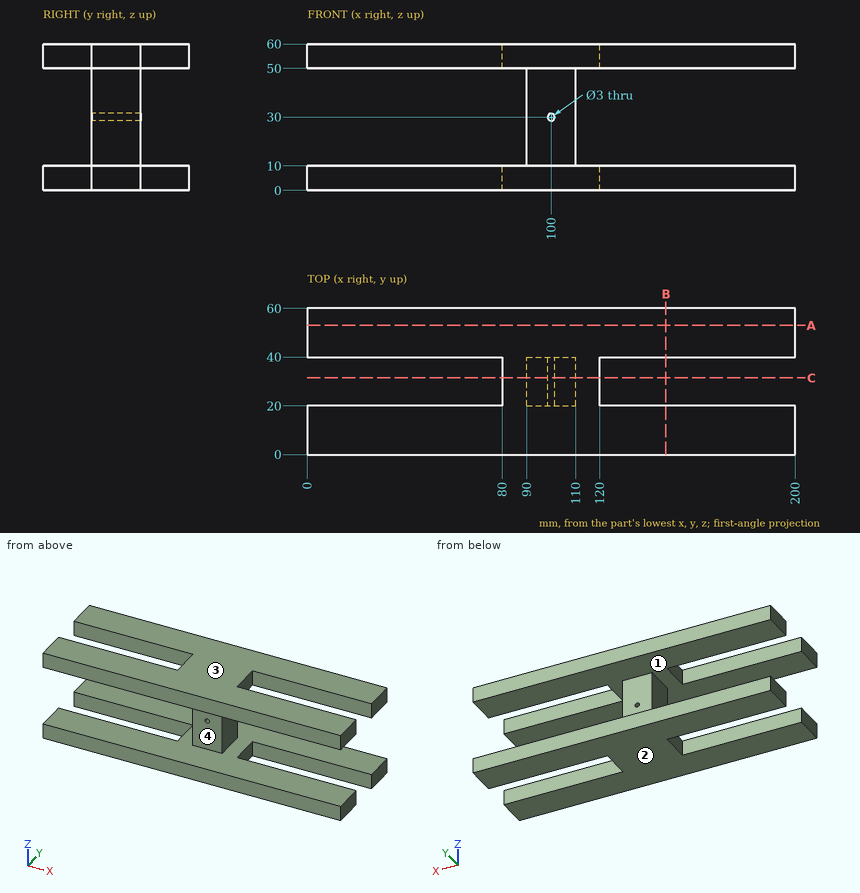
Source: three-view drawing plus pictorial views. Frame: mm from the lowest corner of the part. Give positions to 0.01 mm unless a question says otherwise; leave off trailing zeros. Write each loop counter-clockwise with the first axis right and the second up, starting at its lowest first coordinate (ties: lowest second). Pieces come first, ordered by that corner, then holes. Notation, with made-up numbers: (-16, -34) -> (-2, -34) arc R26 ccw to (-2, -14) -> close; hole circle Ø4 at (42, -33). An arc over 180 degrees is marked (long way). Write item = value, one per line.
Q1. Cut plane C-C on y = 31.5. Return loops of the section in (x, z), then the cut area to 3 significant figures.
Here are the results:
outline = (80, 0) -> (120, 0) -> (120, 10) -> (110, 10) -> (110, 50) -> (120, 50) -> (120, 60) -> (80, 60) -> (80, 50) -> (90, 50) -> (90, 10) -> (80, 10) -> close; hole circle Ø3 at (100, 30)
area = 1,590 mm²
Q2. Line query: line 1 (Z direction, x = 49, y = 52); line 2 (Z direction, x = 100, y = 30.75); line 3 (Y direction, x = 182, z = 51.5). Output: solid intervals per line, ascending. Write a range as from..to.
Here are the results:
line_1 = 0..10, 50..60
line_2 = 0..28.5, 31.5..60
line_3 = 0..20, 40..60
Q3. Cut plane B-B on x = 147. Return loops of the section in (y, z).
Here are the results:
outline = (0, 0) -> (20, 0) -> (20, 10) -> (0, 10) -> close; (0, 50) -> (20, 50) -> (20, 60) -> (0, 60) -> close; (40, 0) -> (60, 0) -> (60, 10) -> (40, 10) -> close; (40, 50) -> (60, 50) -> (60, 60) -> (40, 60) -> close
Q4. First-contact query: pin 1 (3 mm diameter, centred on y = 41, z = 36, fed in from -X); pin 2 (16 mm diameter, centred on y = 25.5, z = 28, fed in from +X); pin 3 (5 mm diameter, centred on y = 31, z = 5, fed in from -X); pin 4 (5 mm diameter, centred on y = 50.5, z = 46.5, fed in from +X). Flat tips, straight axial feed; report the tip coordinate or a pass-through.
Here are the results:
pin_1 = 90
pin_2 = 110
pin_3 = 80
pin_4 = through
Q5. Cut plane A-A on y = 53. Return loops of the section in (x, z).
Here are the results:
outline = (0, 0) -> (200, 0) -> (200, 10) -> (0, 10) -> close; (0, 50) -> (200, 50) -> (200, 60) -> (0, 60) -> close
Q6. Mould query, pull axis Z, two halves, no side actions, for the marked faces 1, 2, 3 and 4. Classes: +Z half, -Z half, draft (parallel to the pull), parting line (faces both ways), or undercut.
Here are the results:
face_1 = undercut
face_2 = -Z half
face_3 = +Z half
face_4 = undercut
